Could you check a few things on this model? Use its own coordinates, in mm. A direction names the side the tool comes from. Round coordinates to 2 decimals unless told otherwise and drop trailing zeros. One line per item, written item: value.
```python
from build123d import *

# Parameters (mm, degrees)
SKETCH1_W                            = 150
SKETCH1_H                            = 80
BOSS_EXTRUDE1_DEPTH                  = 5
SKETCH2_R                            = 6
CUT_EXTRUDE1_DEPTH                   = 5
F_2_3_2_3_DIAMETER_HOLE1_D           = 2.3
F_2_3_2_3_DIAMETER_HOLE1_CSINK_D     = 2.35
F_2_3_2_3_DIAMETER_HOLE1_CSINK_ANGLE = 90
F_3_5_START                          = -1
F_3_5_3_5_DIAMETER_SLOT1_DEPTH       = 7


with BuildPart() as part:
    # Sketch1 → Boss-Extrude1 (new body)
    with BuildSketch(Plane(origin=(0, 0, 0), x_dir=(1, 0, 0), z_dir=(0, 1, 0))):
        Rectangle(SKETCH1_W, SKETCH1_H)
    extrude(amount=BOSS_EXTRUDE1_DEPTH)

    # Sketch2 → Cut-Extrude1 (cut)
    with BuildSketch(Plane(origin=(0, 5, 0), x_dir=(1, 0, 0), z_dir=(0, 1, 0))):
        with Locations(Location((0, 0, 0), (0, 0, 270))):
            Circle(SKETCH2_R)
    extrude(amount=-CUT_EXTRUDE1_DEPTH, mode=Mode.SUBTRACT)

    # Ø2.3 (2.3) Diameter Hole1 (through all)
    with Locations(Plane(origin=(0, 5, 0), x_dir=(1, 0, 0), z_dir=(0, 1, 0))):
        with Locations((18.525219477, 4.313899021), (-12.013304258, 19.048075911), (-12.979283121, 13.346498811), (-9.119541427, 23.344788673), (-5.121281637, 26.028870187), (0, 27.080126555), (4.322325112, 26.34053053), (8.317289006, 24.071257802), (11.39218392, 20.342565819), (12.889434778, 15.772010445), (12.719856903, 11.395868677), (-22.39534299, 1.017693549), (-24.881267093, -4.206895241), (-24.740263888, -10.443726178), (-22.437378406, -15.04431349), (-19.095176636, -18.056881008), (-17.46243869, 4.844417817), (-4.532909997, -17.54299487), (-11.928504706, -20.037357087), (3.910972218, -17.05982561), (8.568273344, -19.524290875), (14.139900873, -19.89356421), (19.874082729, -17.528745152), (23.452077534, -13.540063277), (24.981853962, -9.377653409), (24.881267093, -4.206895241), (23.006620796, 0.176706529)):
            CounterSinkHole(F_2_3_2_3_DIAMETER_HOLE1_D / 2, F_2_3_2_3_DIAMETER_HOLE1_CSINK_D / 2, counter_sink_angle=F_2_3_2_3_DIAMETER_HOLE1_CSINK_ANGLE)

    # Ø3.5 (3.5) Diameter Slot1: read off the stored shape, not the designer's step
    # Ø3.5 (3.5) Diameter Slot1 outline → Ø3.5 (3.5) Diameter Slot1 (cut)
    with BuildSketch(Plane(origin=(0, 0, 0), x_dir=(1, 0, 0), z_dir=(0, 1, 0)).offset(F_3_5_START)):
        with BuildLine():
            Line((41.75, -33.25), (41.75, 33.25))
            ThreePointArc((41.75, 33.25), (40, 35), (38.25, 33.25))
            Line((38.25, 33.25), (38.25, -33.25))
            ThreePointArc((38.25, -33.25), (40, -35), (41.75, -33.25))
        make_face()
        with BuildLine():
            Line((-38.25, -33.25), (-38.25, 33.25))
            ThreePointArc((-38.25, 33.25), (-40, 35), (-41.75, 33.25))
            Line((-41.75, 33.25), (-41.75, -33.25))
            ThreePointArc((-41.75, -33.25), (-40, -35), (-38.25, -33.25))
        make_face()
    extrude(amount=F_3_5_3_5_DIAMETER_SLOT1_DEPTH, mode=Mode.SUBTRACT)

    # 3.5 _3.5_ Diameter Slot1 2: loft between two sections, ruled curve by curve
    f_3_5_3_5_diameter_slot1_2_from = [
        Edge.make_three_point_arc((41.75, 4.975, -33.25), (41.237436867, 4.975, -34.487436867), (40, 4.975, -35)),
        Edge.make_three_point_arc((40, 4.975, -35), (38.762563133, 4.975, -34.487436867), (38.25, 4.975, -33.25)),
        Edge.make_three_point_arc((38.25, 4.975, 33.25), (38.762563133, 4.975, 34.487436867), (40, 4.975, 35)),
        Edge.make_three_point_arc((40, 4.975, 35), (41.237436867, 4.975, 34.487436867), (41.75, 4.975, 33.25)),
        Edge.make_line((38.25, 4.975, -33.25), (38.25, 4.975, 33.25)),
        Edge.make_line((41.75, 4.975, -33.25), (41.75, 4.975, 33.25)),
    ]
    f_3_5_3_5_diameter_slot1_2_to = [
        Edge.make_three_point_arc((41.775, 5, -33.25), (41.255114537, 5, -34.505114537), (40, 5, -35.025)),
        Edge.make_three_point_arc((40, 5, -35.025), (38.744885463, 5, -34.505114537), (38.225, 5, -33.25)),
        Edge.make_three_point_arc((38.225, 5, 33.25), (38.744885463, 5, 34.505114537), (40, 5, 35.025)),
        Edge.make_three_point_arc((40, 5, 35.025), (41.255114537, 5, 34.505114537), (41.775, 5, 33.25)),
        Edge.make_line((38.225, 5, -33.25), (38.225, 5, 33.25)),
        Edge.make_line((41.775, 5, -33.25), (41.775, 5, 33.25)),
    ]
    f_3_5_3_5_diameter_slot1_2 = Solid(Shell([*[Face.make_surface_from_curves(f_3_5_3_5_diameter_slot1_2_from[k], f_3_5_3_5_diameter_slot1_2_to[k]) for k in range(6)], Face(Wire(f_3_5_3_5_diameter_slot1_2_from)), Face(Wire(f_3_5_3_5_diameter_slot1_2_to))]))
    add(f_3_5_3_5_diameter_slot1_2, mode=Mode.SUBTRACT)

    # 3.5 _3.5_ Diameter Slot1 3: loft between two sections, ruled curve by curve
    f_3_5_3_5_diameter_slot1_3_from = [
        Edge.make_three_point_arc((-38.25, 4.975, -33.25), (-38.762563133, 4.975, -34.487436867), (-40, 4.975, -35)),
        Edge.make_three_point_arc((-40, 4.975, -35), (-41.237436867, 4.975, -34.487436867), (-41.75, 4.975, -33.25)),
        Edge.make_three_point_arc((-41.75, 4.975, 33.25), (-41.237436867, 4.975, 34.487436867), (-40, 4.975, 35)),
        Edge.make_three_point_arc((-40, 4.975, 35), (-38.762563133, 4.975, 34.487436867), (-38.25, 4.975, 33.25)),
        Edge.make_line((-41.75, 4.975, -33.25), (-41.75, 4.975, 33.25)),
        Edge.make_line((-38.25, 4.975, -33.25), (-38.25, 4.975, 33.25)),
    ]
    f_3_5_3_5_diameter_slot1_3_to = [
        Edge.make_three_point_arc((-38.225, 5, -33.25), (-38.744885463, 5, -34.505114537), (-40, 5, -35.025)),
        Edge.make_three_point_arc((-40, 5, -35.025), (-41.255114537, 5, -34.505114537), (-41.775, 5, -33.25)),
        Edge.make_three_point_arc((-41.775, 5, 33.25), (-41.255114537, 5, 34.505114537), (-40, 5, 35.025)),
        Edge.make_three_point_arc((-40, 5, 35.025), (-38.744885463, 5, 34.505114537), (-38.225, 5, 33.25)),
        Edge.make_line((-41.775, 5, -33.25), (-41.775, 5, 33.25)),
        Edge.make_line((-38.225, 5, -33.25), (-38.225, 5, 33.25)),
    ]
    f_3_5_3_5_diameter_slot1_3 = Solid(Shell([*[Face.make_surface_from_curves(f_3_5_3_5_diameter_slot1_3_from[k], f_3_5_3_5_diameter_slot1_3_to[k]) for k in range(6)], Face(Wire(f_3_5_3_5_diameter_slot1_3_from)), Face(Wire(f_3_5_3_5_diameter_slot1_3_to))]))
    add(f_3_5_3_5_diameter_slot1_3, mode=Mode.SUBTRACT)


solid = part.part
```
(1) Please list where these lines run through material, in increasing order: L1, parallel to X at y = 2.95, z = 7; L2, parallel to X at y = 0.5, z = 33.5; L3, parallel to Z at x = -23, y = 2.75.
Results below:
L1: x = -75 to -41.75, -38.25 to 38.25, 41.75 to 75
L2: x = -75 to -41.73, -38.27 to 38.27, 41.73 to 75
L3: z = -40 to -2, -0.04 to 14.04, 16.05 to 40
(2) On a 3-axis mill with a long thin cutter (end or side, diameter ignored), from which of +Z, -Z, +X, -X, +Y, -Y can I reach the whole of each face in a straight line? I mean faces 4 (the face through (-75, 2, 1)), 5 (the face through (-41.75, 2, 0)). Say none if no direction works.
Results below:
face 4: +Z, -Z, -X, +Y, -Y
face 5: +Y, -Y
(3) For pin 1 Ø2 at (x, z) = (-12.98, -13.35) entering from -Y, with a flat end and sliding along its axis, tell me the tip position at first contact or that it passes through.
Results below:
pin 1: passes through
(4) We'd pull the mould along Z, two halves only. Please class faces 1 (the face through (-1, 2, -40)), 2 (the face through (-1, 0, 8)), 3 (the face through (-40, 2, 35)): +Z half, -Z half, draft (parallel to the pull), parting line (faces both ways), or undercut.
Results below:
face 1: -Z half
face 2: draft
face 3: undercut
(5) Imagine slicing it at A-A on z = -7.5. Give the number of separate pieces and of enclosed holes in the cut face, then the cut area to 3 significant figures.
Results below:
separate pieces: 3
enclosed holes: 0
area: 715 mm²
